from build123d import *

# Parameters (mm, degrees)
PAD_DEPTH    = 2
PAD001_DEPTH = 2
PAD002_DEPTH = 2


with BuildPart() as part:
    # Sketch → Pad (new body)
    with BuildSketch(Plane.XY):
        with BuildLine():
            ThreePointArc((-27.489858, -0.746794), (27.360019, -2.771163), (-26.781824, 6.243707))
            ThreePointArc((-26.781824, 6.243707), (-26.728683, 3.219003), (-25.249794, 0.579962))
            Line((-25.249794, 0.579962), (-15.435404, -9.800129))
            ThreePointArc((-15.435404, -9.800129), (-14.079498, -9.894335), (-13.873578, -8.55085))
            Line((-13.873578, -8.55085), (-19.209537, -0.614914))
            ThreePointArc((-19.887258, 2.120607), (-19.789586, 0.693092), (-19.209537, -0.614914))
            ThreePointArc((-18.249364, -8.182952), (19.751995, 3.139854), (-19.887258, 2.120607))
            ThreePointArc((-18.249364, -8.182952), (-19.207091, -6.452486), (-20.440588, -4.906446))
            Line((-20.440588, -4.906446), (-25.249794, 0.179962))
            ThreePointArc((-25.249794, 0.179962), (-26.688775, 0.487518), (-27.489858, -0.746794))
        make_face()
    extrude(amount=PAD_DEPTH)

    # Sketch001 → Pad001 (join)
    with BuildSketch(Plane.XY):
        Polygon((19.498872, -43.731184), (9.931054, -26.739808), (-9.567819, -26.530094), (-19.498872, -43.311756), (-9.931054, -60.303132), (9.567819, -60.512846), align=None)
        Polygon((18.5, -43.52147), (9.25, -27.5), (-9.25, -27.5), (-18.5, -43.52147), (-9.25, -59.54294), (9.25, -59.54294), align=None, mode=Mode.SUBTRACT)
    extrude(amount=PAD001_DEPTH)

    # Sketch002 → Pad002 (join)
    with BuildSketch(Plane.XY):
        Polygon((-15.619859, -22.616802), (-19.498872, -43.311756), (-9.567819, -26.530094), (-6.937376, -26.530094), align=None)
        Polygon((19.498872, -43.731184), (15.971505, -22.386626), (6.569976, -26.703659), (9.931054, -26.739808), align=None)
    extrude(amount=PAD002_DEPTH)


solid = part.part
Part model, mm, in its own coordinate system. A direction names the side the tool comes from. Coordinates: 2 decimals unless noted, no trailing zeros. Order: outer loops, then holes, each group sorted by start corner. A loop starts at its lowest first (then second) coordinate and runs counter-clockwise, first axis right, second up.
(1) Slice it at B-B, the plane y = -31. Write the cut outline in (x, z), and give its area (3 significant figures).
Check sheet entries:
outline: (-17.19, 0) - (-11.27, 0) - (-11.27, 2) - (-17.19, 2) - close; (11.27, 0) - (17.39, 0) - (17.39, 2) - (11.27, 2) - close
area: 24.1 mm2
(2) Probe L1, parallel to X at y = 0, z = 0.75; L2, parallel to X at y = -10, z = 1.65; L3, parallel to Y at x = 0, z = 1. List the from-to ranges inside material, lowest first.
Check sheet entries:
L1: x = -27.28 to -25.08, -24.7 to -19.55, 20 to 27.5
L2: x = -25.62 to -17.32, -15.17 to -14.24, 17.32 to 25.62
L3: y = -60.41 to -59.54, -27.5 to -20, 20 to 27.5
(3) Pin check, flat tip, straight feed: pin 1 Ø1 at (x, y) = (19, -12) entering from -Z. Stop position of the tip, or through.
Check sheet entries:
pin 1: stops at z = 0
(4) Slice it at A-A, the plane z = 1.6. State how many separate pieces and enclosed holes the cut face has, and give its area (3 significant figures).
Check sheet entries:
separate pieces: 1
enclosed holes: 2
area: 1,380 mm2
(5) Slice it at D-D, the plane y = 18. Write the cut outline in (x, z).
Check sheet entries:
outline: (-20.79, 0) - (-8.72, 0) - (-8.72, 2) - (-20.79, 2) - close; (8.72, 0) - (20.79, 0) - (20.79, 2) - (8.72, 2) - close
(6) Tool access for faces 4 (the face through (-24.26, -12.95, 0.99)), 5 (the face through (-5, -27.5, 1)), 6 (the face through (-14.4, -9.8, 2)): list every direction of +Z, -Z, +X, -X, +Y, -Y with a clear straight run to the whole face (end or side of a thin tool).
Check sheet entries:
face 4: +Z, -Z, -X
face 5: +Z, -Z
face 6: +Z, +X, -X, +Y, -Y
(7) Pull direction X, two halves, no side cores. Call faces 1 (the face through (-17.534, -32.827, 0.986)), 2 (the face through (14.464, -52.239, 0.986)), 3 (the face through (-13.94, -51.42, 0.99)): pulls with the +X half, pulls with the -X half, needs draft (parallel to the pull), parting line crosses it, or undercut.
Check sheet entries:
face 1: pulls with the -X half
face 2: pulls with the +X half
face 3: undercut
(8) Slice it at C-C, the plane x = 8. Write the cut outline in (y, z).
Check sheet entries:
outline: (-60.5, 0) - (-59.54, 0) - (-59.54, 2) - (-60.5, 2) - close; (-27.5, 0) - (-18.33, 0) - (-18.33, 2) - (-27.5, 2) - close; (18.33, 0) - (26.31, 0) - (26.31, 2) - (18.33, 2) - close
